Geometry: see drawing. Coordinates: mm, zero at the bounding-box minimum. A direction names the side the tool comes from. Give positions to 0.01 mm unless a question says otherwise; leave off trailing zeros. Write each loop counter-clockwise with the first axis right and the second up, starting at its lowest first coordinate (ties: lowest second). Pieces come first, ordered by that corner, then holes.
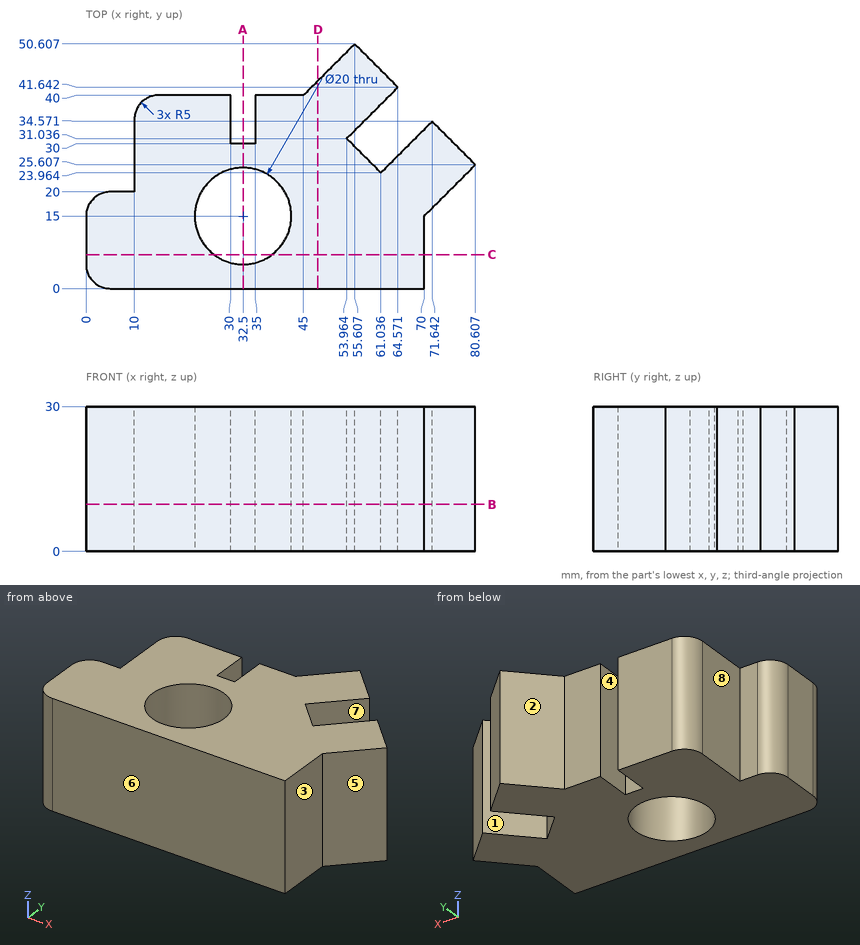
Q1. Material intervals for line 1 along Y through (x, z) = (32.5, 24); line 2 along X through (y, z) = (38.5, 12.75); line 3 along X through (y, z) = (12.5, 19), sorted ascending.
Q2. Mould query, pull axis Y, two halves, no side actions, for the marked faces 1, 2 and 3. Classes: +Y half, -Y half, draft (parallel to the pull), parting line (faces both ways), or undercut.
Q3. Access query for the marked faces 4, 5, 6, 7 and 8. Directions: +Z, -Z, +X, -X, +Y, -Y. A direction counts if a zero-diameter tool reaches every point of the face in a straight line with its end or side. Return the directions, or none.
Q4. Section D-D, the plane x = 48. Return the cut outline in (y, z), then the cut area to 3 significant figures.
Q5. Pin query (flat end, axial travel): pin 1 (2 mm diameter, centred on y = 40, z = 9, fed in from -X); pin 2 (12 mm diameter, centred on x = 11, z = 8.5, fed in from +Y); pin 3 (7.5 mm diameter, centred on y = 29.5, z = 21.5, fed in from -X). Return the tip coordinate at first contact, or that it passes through.
Q6. Section B-B, the plane z = 9.75. Return the cut outline in (x, y) (1 decimal), then the cut area to 3 significant figures.
Q7. Section A-A, the plane x = 32.5. Return the cut outline in (y, z), then the cut area to 3 significant figures.
Q8. Section C-C, the plane y = 7. Return the cut outline in (x, z), then the cut area to 3 significant figures.
Solutions:
1. line 1: y = 0 to 5, 25 to 30
1. line 2: x = 11.43 to 30, 35 to 61.43
1. line 3: x = 0 to 22.82, 42.18 to 70
2. face 1: undercut
2. face 2: +Y half
2. face 3: draft
3. face 4: +Z, -Z, +Y
3. face 5: +Z, -Z, +X, -Y
3. face 6: +Z, -Z, +X, -X, -Y
3. face 7: +Z, -Z
3. face 8: +Z, -Z, -X, +Y
4. outline: (0, 0) - (43, 0) - (43, 30) - (0, 30) - close
4. area: 1,290 mm2
5. pin 1: stops at x = 12
5. pin 2: stops at y = 40
5. pin 3: stops at x = 10
6. outline: (0, 5) arc R5 ccw to (5, 0) - (70, 0) - (70, 15) - (80.6, 25.6) - (71.6, 34.6) - (61, 24) - (54, 31) - (64.6, 41.6) - (55.6, 50.6) - (45, 40) - (35, 40) - (35, 30) - (30, 30) - (30, 40) - (15, 40) arc R5 ccw to (10, 35) - (10, 20) - (5, 20) arc R5 ccw to (0, 15) - close; hole circle Ø20 at (32.5, 15)
6. area: 2,290 mm2
7. outline: (0, 0) - (5, 0) - (5, 30) - (0, 30) - close; (25, 0) - (30, 0) - (30, 30) - (25, 30) - close
7. area: 300 mm2
8. outline: (0, 0) - (26.5, 0) - (26.5, 30) - (0, 30) - close; (38.5, 0) - (70, 0) - (70, 30) - (38.5, 30) - close
8. area: 1,740 mm2
